Could you check a few things on this model? Use its own coordinates, in mm. A direction names the side the tool comes from. Round coordinates to 2 decimals unless told otherwise and drop trailing zeros. Loops run counter-clockwise (first coordinate to the right, second up) from the corner with the lowest first, then second, coordinate; pieces in that order, holes last. Notation, with made-up numbers: (3.5, 56.5) -> (58.5, 56.5) arc R27 cw to (58.5, 83.5) -> close; hole circle Ø8 at (81.25, 7). An arc over 180 degrees is marked (long way). Write each question's results on one line, items separated by ' | '.
from build123d import *
from OCP.BRepFilletAPI import BRepFilletAPI_MakeChamfer

# Parameters (mm, degrees)
SKETCH_1_W       = 14.75
SKETCH_1_H       = 20.67
EXTRUDE_1_DEPTH  = 1.28
EXTRUDE_2_DEPTH  = 3
CHAMFER_3_SIZE   = 2
CHAMFER_3_SIZE_2 = 11.342563639
CHAMFER_4_SIZE   = 0.5
CHAMFER_4_SIZE2  = 0.288675135
CHAMFER_5_SIZE   = 3
CHAMFER_5_SIZE_2 = 1.041889066
CHAMFER_6_SIZE   = 0.978668112
CHAMFER_6_SIZE_2 = 9
SKETCH_3_W       = 11.74
SKETCH_3_H       = 18.5
EXTRUDE_3_DEPTH  = 7.96


with BuildPart() as part:
    # 草图1 → 凸台-拉伸1 (new body)
    with BuildSketch(Plane.XY):
        Rectangle(SKETCH_1_W, SKETCH_1_H)
    extrude(amount=EXTRUDE_1_DEPTH)

    # 草图2 → 凸台-拉伸2 (add)
    with BuildSketch(Plane.XY.offset(1.28)):
        Polygon((0, -4.8), (-3, -4.8), (-3, 4.8), (3, 4.8), (3, -4.8), align=None)
    extrude(amount=EXTRUDE_2_DEPTH)

    # 倒角3
    # the kernel refuses this chamfer: 11.342563639, 2 mm, written as the material it takes off along each edge
    with BuildSketch(Plane(origin=(32.474091667, -4.8, 4.28), x_dir=(0, -0.21013876076743543, -0.9776715712462578), z_dir=(-1, 0, 0))) as chamfer_3_piece_1:
        Polygon((CHAMFER_3_SIZE * 0.977671571246, -CHAMFER_3_SIZE * 0.210138760767), (-CHAMFER_3_SIZE_2 * 0.210138760772, -CHAMFER_3_SIZE_2 * 0.977671571267), (0, 0), align=None)
    extrude(amount=64.948183335, mode=Mode.SUBTRACT)

    # 倒角4: one chamfer whose edges measure the first distance from different faces: ONE call of the kernel's chamfer builder (chamfer() names one face for all edges)
    chamfer_4_edges_1 = [part.edges().sort_by_distance(p)[0] for p in [
        (7.375, 0, 1.28),
    ]]
    chamfer_4_side_1 = [part.faces().sort_by_distance(p)[0] for p in [
        (7.375, 0, 0.64),
    ]]
    chamfer_4_edges_2 = [part.edges().sort_by_distance(p)[0] for p in [
        (0, 10.335, 1.28),
    ]]
    chamfer_4_side_2 = [part.faces().sort_by_distance(p)[0] for p in [
        (0, 10.335, 0.64),
    ]]
    chamfer_4_edges_3 = [part.edges().sort_by_distance(p)[0] for p in [
        (-7.375, 0, 1.28),
    ]]
    chamfer_4_side_3 = [part.faces().sort_by_distance(p)[0] for p in [
        (-7.375, 0, 0.64),
    ]]
    chamfer_4_edges_4 = [part.edges().sort_by_distance(p)[0] for p in [
        (0, -10.335, 1.28),
    ]]
    chamfer_4_side_4 = [part.faces().sort_by_distance(p)[0] for p in [
        (0, -10.335, 0.64),
    ]]
    chamfer_4 = BRepFilletAPI_MakeChamfer(part.part.solid().wrapped)
    for e in chamfer_4_edges_1:
        chamfer_4.Add(CHAMFER_4_SIZE, CHAMFER_4_SIZE2, e.wrapped, chamfer_4_side_1[0].wrapped)  # the first distance lies on this face
    for e in chamfer_4_edges_2:
        chamfer_4.Add(CHAMFER_4_SIZE, CHAMFER_4_SIZE2, e.wrapped, chamfer_4_side_2[0].wrapped)  # the first distance lies on this face
    for e in chamfer_4_edges_3:
        chamfer_4.Add(CHAMFER_4_SIZE, CHAMFER_4_SIZE2, e.wrapped, chamfer_4_side_3[0].wrapped)  # the first distance lies on this face
    for e in chamfer_4_edges_4:
        chamfer_4.Add(CHAMFER_4_SIZE, CHAMFER_4_SIZE2, e.wrapped, chamfer_4_side_4[0].wrapped)  # the first distance lies on this face
    add(Compound.cast(chamfer_4.Shape()), mode=Mode.REPLACE)

    # 倒角5
    # the kernel refuses this chamfer: 3, 1.041889066 mm, written as the material it takes off along each edge
    with BuildSketch(Plane(origin=(10.782584198, 4.8, 3.972739015), x_dir=(0, 0.013184058198646008, -0.9999130865277315), z_dir=(-1, 0, 0))) as chamfer_5_piece_1_section:
        Polygon((CHAMFER_5_SIZE * 0.999913086528, CHAMFER_5_SIZE * 0.0131840581986), (CHAMFER_5_SIZE_2 * 0.160649322571, CHAMFER_5_SIZE_2 * 0.987011547633), (0, 0), align=None)
    chamfer_5_piece_1 = extrude(amount=21.565168395, mode=Mode.PRIVATE)
    chamfer_5_piece_1 = split(chamfer_5_piece_1, bisect_by=Plane(origin=(0, 4.454539571, 1.28), z_dir=(0, 0, 1)), keep=Keep.TOP, mode=Mode.PRIVATE)
    add(chamfer_5_piece_1, mode=Mode.SUBTRACT)

    # 倒角6
    # the kernel refuses this chamfer: 9, 0.978668112 mm, written as the material it takes off along each edge
    with BuildSketch(Plane(origin=(26.395258852, -4.8, 2.28), x_dir=(0, -0.30567862025886394, -0.952134749453373), z_dir=(-1, 0, 0))) as chamfer_6_piece_1:
        Polygon((CHAMFER_6_SIZE * 0.952134749764, -CHAMFER_6_SIZE * 0.305678620359), (-CHAMFER_6_SIZE_2 * 0.466371139297, -CHAMFER_6_SIZE_2 * 0.884589147814), (0, 0), align=None)
    extrude(amount=52.790517704, mode=Mode.SUBTRACT)

    # 草图3 → 凸台-拉伸3 (add)
    with BuildSketch(Plane(origin=(0, 0, 0), x_dir=(-1, 0, 0), z_dir=(0, 0, -1))):
        Rectangle(SKETCH_3_W, SKETCH_3_H)
    extrude(amount=EXTRUDE_3_DEPTH)


solid = part.part
1) I want a section at B-B, the plane y = -7.5. Write out the boundary of the cut face in (x, z) (3 decimals).
Model answer:
outline: (-7.375, 0) -> (-5.87, 0) -> (-5.87, -7.96) -> (5.87, -7.96) -> (5.87, 0) -> (7.375, 0) -> (7.375, 0.78) -> (7.086, 1.28) -> (-7.086, 1.28) -> (-7.375, 0.78) -> close
2) I want a section at D-D, the plane x = -0.75. Write out the boundary of the cut face in (y, z) (3 decimals), plus the area to 3 significant figures.
Model answer:
outline: (-10.335, 0) -> (-9.25, 0) -> (-9.25, -7.96) -> (9.25, -7.96) -> (9.25, 0) -> (10.335, 0) -> (10.335, 0.78) -> (10.046, 1.28) -> (4.688, 1.28) -> (3.784, 3.763) -> (-4.8, 1.301) -> (-4.8, 1.28) -> (-10.046, 1.28) -> (-10.335, 0.78) -> close | area: 185 mm2
3) I want a section at A-A, the plane x = 3.75. Write out the boundary of the cut face in (y, z) (3 decimals), plus the area to 3 significant figures.
Model answer:
outline: (-10.335, 0) -> (-9.25, 0) -> (-9.25, -7.96) -> (9.25, -7.96) -> (9.25, 0) -> (10.335, 0) -> (10.335, 0.78) -> (10.046, 1.28) -> (-10.046, 1.28) -> (-10.335, 0.78) -> close | area: 174 mm2
4) I need wall thicknesses on line 1 (X direction, y = 4.25, z = -0.5); line 2 (Y direction, x = -0.25, z = -5.5); line 3 (Z direction, x = 5, y = 8). Which ranges of each line are inside material? Lowest first, please.
Model answer:
line 1: x = -5.87 to 5.87 | line 2: y = -9.25 to 9.25 | line 3: z = -7.96 to 1.28
5) I want a section at C-C, the plane z = -4.5. Write out the boundary of the cut face in (x, y), plus the area to 3 significant figures.
Model answer:
outline: (-5.87, -9.25) -> (5.87, -9.25) -> (5.87, 9.25) -> (-5.87, 9.25) -> close | area: 217 mm2
6) I'm going to push flat-ended pins straight in: pin 1 (2.5 mm diameter, centred on y = 2, z = 3, fed in from +X); pin 2 (2.5 mm diameter, centred on y = 0.5, z = -5, fed in from -X); pin 3 (4 mm diameter, centred on x = 2, z = -2.5, fed in from -Y). Where does each tip first touch, or does it pass through?
Model answer:
pin 1: stops at x = 3 | pin 2: stops at x = -5.87 | pin 3: stops at y = -9.25
7) For faces 1 (the flat face through (-3, 1, 2)), 2 (the flat face through (5.87, 0, -4)), 3 (the flat face through (0, -9.25, -4)), 4 (the flat face through (3, 1, 2)), 5 (the flat face through (-5.87, 0, -4)), which set-ups out of +Z, -Z, +X, -X, +Y, -Y let a thin tool reach every point of the face, with its end or its side?
Model answer:
face 1: +Z, -X, +Y, -Y | face 2: -Z, +X, +Y, -Y | face 3: -Z, +X, -X, -Y | face 4: +Z, +X, +Y, -Y | face 5: -Z, -X, +Y, -Y
